Input: dimensioned drawing with shaded views. Units: mm. Origin: part minimum x, y, z. Give positions to 0.01 mm unless a question says otherwise; leave off trailing zeros. Write each loop counter-clockwise with the first axis right and the second up, starting at its lowest first coordinate (ties: lowest second). Pieces come first, ordered by that corner, then holes. Notation, with made-up numbers: (-17.75, 18.25) -> (22.25, 18.25) arc R11 ccw to (22.25, 28.25) -> close; hole circle Ø10 at (41, 57.25). An arc over 180 degrees is marked (long way). Answer as a JSON object with one key per item and string values. Group by question number.
(1) Section query C-C on z = 3. Output: boundary loops of the cut face in (x, y).
(2) Section query D-D on y = 51. Output: boundary loops of the cut face in (x, z), plus the area to 3 significant figures.
(3) Section query B-B on y = 36. Output: boundary loops of the cut face in (x, z).
(4) Contact query for a flat-ended pin moving along its axis: pin 1 Ø1 at (y, z) = (25, 3) entering from -X. Output: stop coordinate, or through.
(5) Material intervals for probe 1 along X at (y, z) = (20, 0.75); probe 2 along X at (y, z) = (28.5, 4.5); probe 3 along Y at (x, z) = (13, 4.5), sorted ascending.
(6) Section query A-A on x = 38. Output: boundary loops of the cut face in (y, z), plus the area to 3 significant figures.
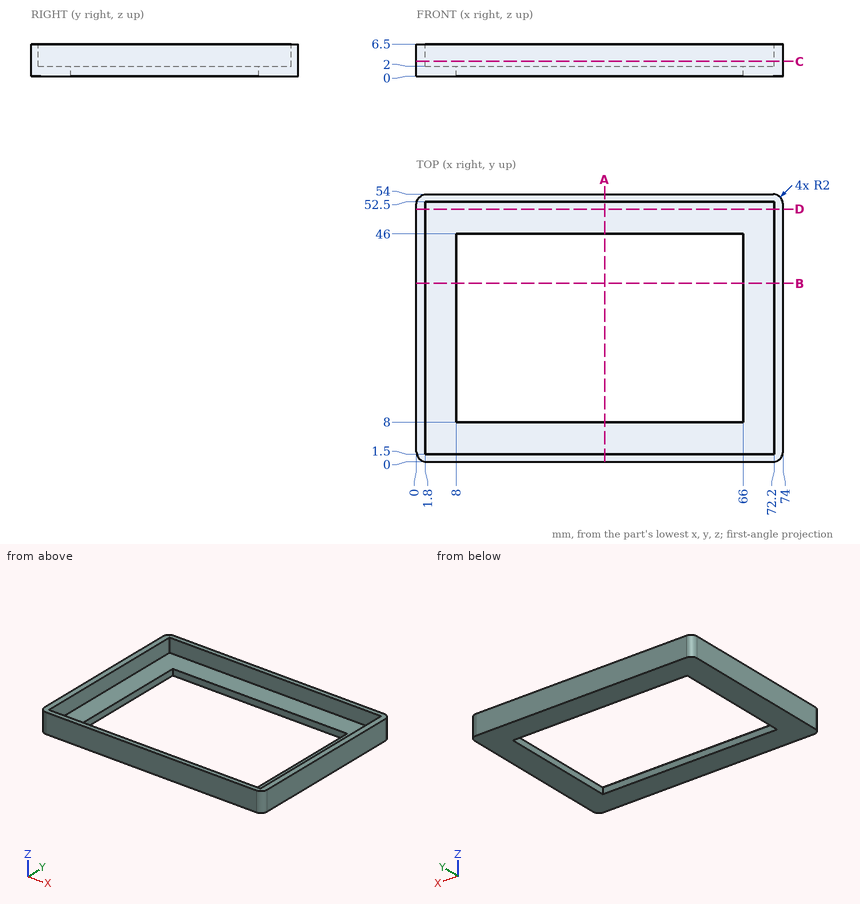
Answer list:
{
 "1": {"outline": "(0, 2) arc R2 ccw to (2, 0) -> (72, 0) arc R2 ccw to (74, 2) -> (74, 52) arc R2 ccw to (72, 54) -> (2, 54) arc R2 ccw to (0, 52) -> close; hole (1.8, 1.5) -> (72.2, 1.5) -> (72.2, 52.5) -> (1.8, 52.5) -> close"},
 "2": {"outline": "(0, 0) -> (74, 0) -> (74, 6.5) -> (72.2, 6.5) -> (72.2, 2) -> (1.8, 2) -> (1.8, 6.5) -> (0, 6.5) -> close", "area": "164 mm2"},
 "3": {"outline": "(0, 0) -> (8, 0) -> (8, 2) -> (1.8, 2) -> (1.8, 6.5) -> (0, 6.5) -> close; (66, 0) -> (74, 0) -> (74, 6.5) -> (72.2, 6.5) -> (72.2, 2) -> (66, 2) -> close"},
 "4": {"pin 1": "x = 0"},
 "5": {"probe 1": "0 to 8, 66 to 74", "probe 2": "0 to 1.8, 72.2 to 74", "probe 3": "0 to 1.5, 52.5 to 54"},
 "6": {"outline": "(0, 0) -> (8, 0) -> (8, 2) -> (1.5, 2) -> (1.5, 6.5) -> (0, 6.5) -> close; (46, 0) -> (54, 0) -> (54, 6.5) -> (52.5, 6.5) -> (52.5, 2) -> (46, 2) -> close", "area": "45.5 mm2"}
}
